Source: CAD feature listing. Evaluate the final solid. Frame: model axes, mm. A direction names the side the tool comes from. Coordinates: 2 decimals unless noted, no trailing zeros. Order: outer loops, then holes, each group sorted by start corner. A loop starts at its lowest first (then second) coordinate and runs counter-clockwise, first axis right, second up. Notation, with made-up numbers: (-28, 76) -> (-9, 76) arc R27 cw to (-9, 107) -> close; hole circle Ø4 at (-36, -8.75). An arc over 180 degrees is marked (long way). Write item = value, one per line. Start each with the question number.
Item 1: Mould query, pull axis Y, two halves, no side actions, for faces 1 (the flat face through (165.714, -17.911, 30.882)), 2 (the flat face through (332.5, -0.2, -5.2)), 3 (the cylindrical face through (307.85, -3.604, -11.446)). Classes: released by +Y, released by -Y, zero draft, split by the parting line, or undercut.
Item 2: Section query B-B (x = 269.5). Output: boundary loops of the cut face in (y, z).
Item 3: Set-up query: faces 4 (the flat face through (0, 0, 0)), 5 (the flat face through (69, -10, 2)), 6 (the flat face through (166, 0, -35.7)). Return all of +Z, -Z, +X, -X, +Y, -Y with unobstructed straight access to the full face (end or side cutting, diameter ignored); none if empty.
Item 4: Ray query, line 1 along Y through (x, z) = (133.5, 14); line 2 along X through (y, z) = (22, 19.5); line 3 along X through (y, z) = (0, 7). Return the intervals inside material, ascending. Write a range as [from, to].
Item 5: Contact query for flat-ended pins moving along their axis: pin 1 (4 mm diameter, centred on x = 151.5, y = -7, fed in from -Z); pin 2 (1.5 mm diameter, centred on x = 299, y = 14, fed in from -Z); pin 3 (1.5 mm diameter, centred on y = -12, z = -7.5, fed in from -X); pin 4 (5 mm diameter, centred on x = 174, y = 1, fed in from -Z). Output: stop coordinate, or through.
Item 6: Section query A-A (x = 316.5). Output: boundary loops of the cut face in (y, z).
```python
from build123d import *

# Parameters (mm, degrees)
CUT_EXTRUDE2_DEPTH = 102
CIRPATTERN2_COUNT  = 12


with BuildPart() as part:
    # Sketch1 → Revolve1 (revolve)
    with BuildSketch(Plane.XY, mode=Mode.PRIVATE) as revolve1_sk:
        Polygon((0, 0), (0, 5), (15, 5), (15, 10), (69, 10), (69, 12.2), (105, 12.2), (105, 38.2), (225, 38.2), (225, 15), (251.5, 15), (251.5, 12.5), (282.5, 12.5), (282.5, 12), (332.5, 12), (332.5, 5), (347.5, 5), (347.5, 0), align=None)
    revolve(revolve1_sk.sketch.rotate(Axis((347.5, 0, 0), (-1, 0, 0)), 90), axis=Axis((347.5, 0, 0), (-1, 0, 0)))  # turned: the seam where the file's is

    # Sketch2 → Cut-Extrude2 (cut)
    with BuildSketch(Plane(origin=(216, 0, 0), x_dir=(0, 0, -1), z_dir=(1, 0, 0))):
        Polygon((38.2, 0), (38.2, 5), (35.7, 5), (35.7, -5), (38.2, -5), align=None)
    cut_extrude2 = extrude(amount=-CUT_EXTRUDE2_DEPTH, mode=Mode.SUBTRACT)

    # CirPattern2: Cut-Extrude2 ×12 about axis
    cirpattern2_axis = Axis((0, 0, 0), (1, 0, 0))
    for i in range(1, CIRPATTERN2_COUNT):
        add(cut_extrude2.rotate(cirpattern2_axis, i * 360 / CIRPATTERN2_COUNT), mode=Mode.SUBTRACT)


solid = part.part
```
Computed:
q1.face_1 = undercut
q1.face_2 = zero draft
q1.face_3 = split by the parting line
q2.outline = circle Ø25 at (0, 0)
q3.face_4 = +Z, -Z, -X, +Y, -Y
q3.face_5 = -X
q3.face_6 = -Z
q4.line_1 = [-35.54, -34.25], [-33.14, 33.14], [34.25, 35.54]
q4.line_2 = [105, 225]
q4.line_3 = [15, 332.5]
q5.pin_1 = -37.87
q5.pin_2 = through
q5.pin_3 = 105
q5.pin_4 = -35.7
q6.outline = circle Ø24 at (0, 0)
